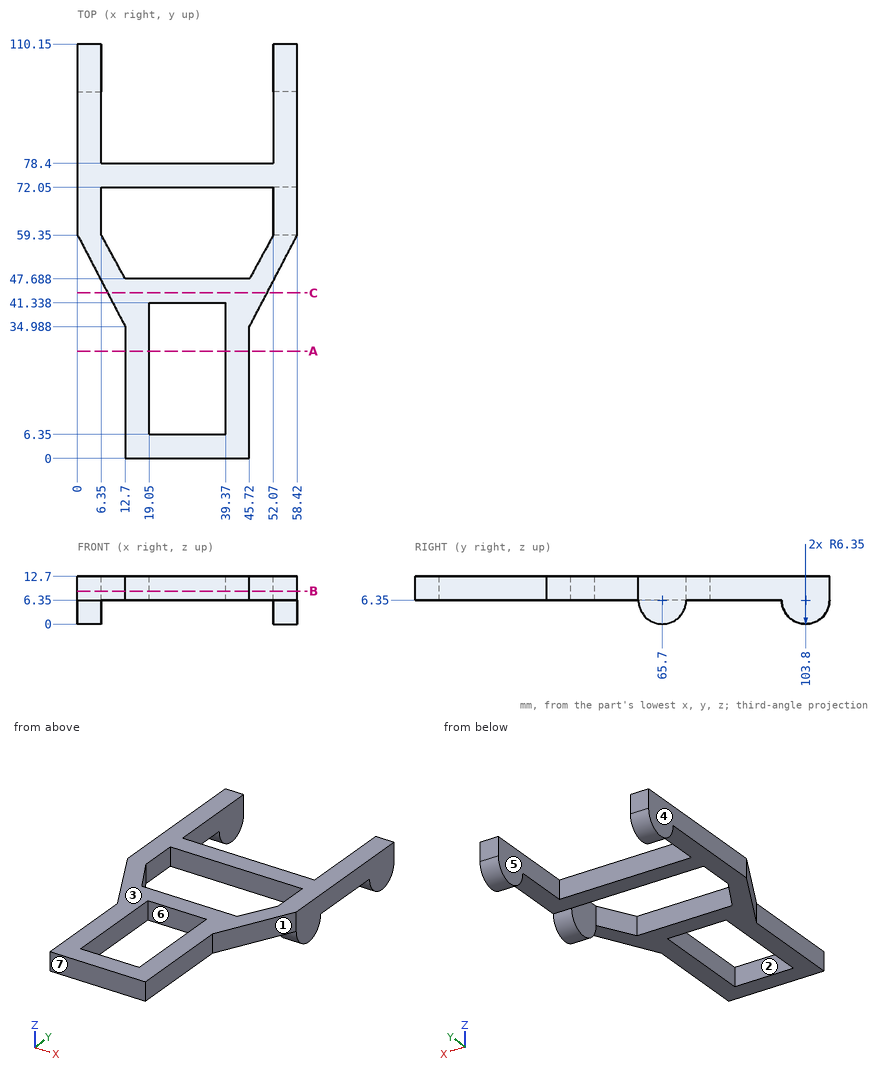
Part print with two shaded views. Sizes in mm from the minimum x, y, z corner. A direction names the side the tool comes from. Give positions to 0.01 mm unless a question says otherwise; leave off trailing zeros. Order: outer loops, then holes, each group sorted by start corner. A loop starts at its lowest first (then second) coordinate and runs counter-clockwise, first axis right, second up. Notation, with made-up numbers: M -14,17 L 15,17 A17 ccw 15,39 Z; hole C 32,31 d4. An arc over 180 degrees is marked long. Write item = value, one per line.
Q1. Cut at C-C, the plane y = 44. List the corners of the cut face in (x, z).
Derived:
outline = M 8,6.35 L 50.42,6.35 L 50.42,12.7 L 8,12.7 Z
Q2. Cut at B-B, the plane z = 8.75. List the corners of the cut face in (x, y).
Derived:
outline = M 0,59.35 L 12.7,34.99 L 12.7,0 L 45.72,0 L 45.72,34.99 L 58.42,59.35 L 58.42,110.15 L 52.07,110.15 L 52.07,78.4 L 6.35,78.4 L 6.35,110.15 L 0,110.15 Z; hole M 6.35,59.35 L 12.7,47.69 L 45.72,47.69 L 52.07,59.35 L 52.07,72.05 L 6.35,72.05 Z; hole M 19.05,6.35 L 39.37,6.35 L 39.37,41.34 L 19.05,41.34 Z
Q3. Flat gauge pins, fed straight in: pin 1 (1 mm diameter, centred on y = 56.5, z = 4.5, fed in from -X); pin 2 (7 mm diameter, centred on y = 27, z = 8.5, fed in from -X); pin 3 (1.9 mm diameter, centred on y = 20.5, z = 10.5, fed in from +X); pin 4 (1.9 mm diameter, centred on x = 27.5, z = 9.5, fed in from +Y). Where does each tip first touch, or does it go through?
Derived:
pin_1 = through
pin_2 = 12.7
pin_3 = 45.72
pin_4 = 78.4
Q4. Tool access for the marked faces 5, 6 and 7: list every direction of +Z, -Z, +X, -X, +Y, -Y with a clear straight run to the whole face (end or side of a thin tool).
Derived:
face_5 = +Z, -Z, +Y
face_6 = +Z, -Z
face_7 = +Z, -Z, +X, -X, -Y
Q5. Cut at A-A, the plane y = 28.5. List the corners of the cut face in (x, z).
Derived:
outline = M 12.7,6.35 L 19.05,6.35 L 19.05,12.7 L 12.7,12.7 Z; M 39.37,6.35 L 45.72,6.35 L 45.72,12.7 L 39.37,12.7 Z
Q6. Two-plate mould, pull along X, no slides. Class the marked faces 1, 2, 3 and 4: pulls with the +X half, pulls with the -X half, needs draft (parallel to the pull), parting line crosses it, or undercut.
Derived:
face_1 = pulls with the +X half
face_2 = undercut
face_3 = needs draft
face_4 = pulls with the -X half
Q7. Drill centre lines: line 1 (Y direction, x = 38.5, z = 8); line 2 (X direction, y = 27, z = 8.75); line 3 (X direction, y = 66.5, z = 6.5). Where is each one in solid material? Low to high. Write a range as [from, to].
Derived:
line_1 = [0, 6.35], [41.34, 47.69], [72.05, 78.4]
line_2 = [12.7, 19.05], [39.37, 45.72]
line_3 = [0, 6.35], [52.07, 58.42]
